from build123d import *

# Parameters (mm, degrees)
F1_DEPTH = 26.924
F2_W     = 47.987626
F2_H     = 46.88446
F3_DEPTH = 6.35


with BuildPart() as f1:
    # F0 (on Right) → F1 (new body, symmetric)
    with BuildSketch(Plane.YZ):
        with BuildLine():
            Line((-64.30237, 9.54966), (-64.30237, -8.503878))
            Line((-64.30237, -8.503878), (-57.232525, -8.503878))
            add(Edge.make_bspline(
                [(-57.232525, -8.503878), (-53.551972, 6.674868), (-35.007033, 5.623281), (-32.202799, -8.503878)],
                knots=[0, 0, 0, 0, 25.029726, 25.029726, 25.029726, 25.029726], degree=3))
            Line((-32.202799, -8.503878), (23.917472, -8.503878))
            add(Edge.make_bspline(
                [(33.688288, 5.422598), (26.724873, 4.578994), (23.683522, -1.269759), (23.917472, -8.503878)],
                knots=[0, 0, 0, 0, 17.012219, 17.012219, 17.012219, 17.012219], degree=3))
            Line((33.688288, 5.422598), (62.469676, 5.422598))
            add(Edge.make_bspline(
                [(62.469676, 5.422598), (71.99423, 4.812944), (74.216753, -2.20556), (74.167915, -8.503878)],
                knots=[0, 0, 0, 0, 18.187785, 18.187785, 18.187785, 18.187785], degree=3))
            Line((74.167915, -8.503878), (79.810925, -8.503878))
            Line((79.810925, -8.503878), (79.810925, 15.866313))
            Line((79.810925, 15.866313), (26.938191, 15.866313))
            Line((26.938191, 15.866313), (22.025237, 25.458271))
            Line((22.025237, 25.458271), (0, 25.458271))
            Line((0, 25.458271), (-32.017246, 12.357062))
            Line((-32.017246, 12.357062), (-64.30237, 9.54966))
        make_face()
    extrude(amount=F1_DEPTH, both=True)

    # F2 (on face) → F3 (cut)
    with BuildSketch(Plane.XY.offset(15.866313)):
        with Locations((-0.038729, 53.329439)):
            Rectangle(F2_W, F2_H)
    extrude(amount=-F3_DEPTH, mode=Mode.SUBTRACT)


solid = f1.part
Input: part model. Units: mm. Frame: model coordinates. A direction names the side the tool comes from. Give positions to 0.01 mm unless a question says otherwise; leave off trailing zeros. Order: outer loops, then holes, each group sorted by start corner. A loop starts at its lowest first (then second) coordinate and runs counter-clockwise, first axis right, second up. Notation, with made-up numbers: (-16.75, -25) -> (13.25, -25) arc R23 cw to (13.25, -11) -> close; hole circle Ø4 at (40.25, 87.5). An arc over 180 degrees is marked (long way). Use one line per item in the form item = value.
1) Section C-C, the plane y = -2.5. Return loops of the section in (x, z), and give its area (3 significant figures).
Response values:
outline = (-26.92, -8.5) -> (26.92, -8.5) -> (26.92, 24.44) -> (-26.92, 24.44) -> close
area = 1,770 mm^2
2) Mould query, pull axis X, two halves, no side actions, for faces 1 (the flat face through (-26.924, 7, 9)), 2 (the flat face through (-24.033, 53, 13)), 3 (the flat face through (0, -5, -8.504)). Classes: pulls with the +X half, pulls with the -X half, needs draft (parallel to the pull), parting line crosses it, or undercut.
Response values:
face_1 = pulls with the -X half
face_2 = undercut
face_3 = needs draft
3) First-contact query: pin 1 Ø1.5 at (x, y) = (-0.5, -12) entering from +Z; pin 2 Ø14 at (x, y) = (7, 64) entering from +Z; pin 3 Ø4 at (x, z) = (18.5, 18) entering from -Y. Flat tips, straight axial feed; report the tip coordinate or a pass-through.
Response values:
pin_1 = 20.85
pin_2 = 9.52
pin_3 = -23.11
4) Section B-B, the plane z = -0.5. Count the separate pieces of the cut face and the enclosed holes in it, and give its area (3 significant figures).
Response values:
separate_pieces = 3
enclosed_holes = 0
area = 4,360 mm^2
5) Section A-A, the plane y = 49.5. Return loops of the section in (x, z).
Response values:
outline = (-26.92, 5.42) -> (26.92, 5.42) -> (26.92, 15.87) -> (23.96, 15.87) -> (23.96, 9.52) -> (-24.03, 9.52) -> (-24.03, 15.87) -> (-26.92, 15.87) -> close
6) Reachability of faces 4 (the flat face through (0, 48, 5.423)), 5 (the flat face through (0, 29.887, 13)), 6 (the flat face through (4, 77, 15.866)) from +Z, -Z, +X, -X, +Y, -Y: full face, straight path, thin tool, end or side. Return the list, or none.
Response values:
face_4 = -Z, +X, -X
face_5 = +Z
face_6 = +Z, +X, -X, +Y
7) Line query: probe 1 along X at (y, z) = (71.5, 10.5); probe 2 along Y at (x, z) = (-5, -1.5); probe 3 along Y at (x, z) = (-13, -7). Output: solid intervals per line, ascending.
Response values:
probe_1 = -26.92 to -24.03, 23.96 to 26.92
probe_2 = -64.3 to -53.65, -35.64 to 24.93, 73 to 79.81
probe_3 = -64.3 to -56.8, -32.57 to 23.92, 74.13 to 79.81
